```python
from build123d import *

# Parameters (mm, degrees)
PAD008_DEPTH = 2.8
FILLET001_R  = 0.4
POCKET_DEPTH = 2.801


with BuildPart() as part:
    # Sketch008 (on Face4 of ShapeBinder007) → Pad008 (new body)
    with BuildSketch(Plane(origin=(0, 20.1, 0), x_dir=(-1, 0, 0), z_dir=(0, 1, 0))):
        with BuildLine():
            Line((37.8, 63.2), (37.8, 60.4))
            Line((37.8, 60.4), (23.8, 60.4))
            ThreePointArc((23.8, 60.4), (23.4, 60), (23.8, 59.6))
            Line((23.8, 59.6), (37.8, 59.6))
            Line((37.8, 59.6), (37.8, -33.8))
            Line((37.8, -33.8), (23.8, -33.8))
            ThreePointArc((23.8, -33.8), (23.4, -34.2), (23.8, -34.6))
            Line((23.8, -34.6), (37.8, -34.6))
            Line((37.8, -34.6), (37.8, -37.4))
            Line((37.8, -37.4), (35.8, -38.15))
            Line((35.8, -38.15), (35.8, -37.4))
            Line((35.8, -37.4), (33, -37.4))
            Line((33, -39.4), (33, -37.4))
            Line((25.535898, -37.4), (33, -39.4))
            Line((-25.535898, -37.4), (25.535898, -37.4))
            Line((-33, -39.4), (-25.535898, -37.4))
            Line((-33, -37.4), (-33, -39.4))
            Line((-35.8, -37.4), (-33, -37.4))
            Line((-35.8, -38.15), (-35.8, -37.4))
            Line((-37.8, -37.4), (-35.8, -38.15))
            Line((-37.8, -37.4), (-37.8, -34.6))
            Line((-37.8, -34.6), (-23.8, -34.6))
            ThreePointArc((-23.8, -34.6), (-23.4, -34.2), (-23.8, -33.8))
            Line((-23.8, -33.8), (-37.8, -33.8))
            Line((-37.8, -33.8), (-37.8, 59.6))
            Line((-23.8, 59.6), (-37.8, 59.6))
            ThreePointArc((-23.8, 59.6), (-23.4, 60), (-23.8, 60.4))
            Line((-37.8, 60.4), (-23.8, 60.4))
            Line((-37.8, 60.4), (-37.8, 63.2))
            Line((-37.8, 63.2), (-35.8, 63.95))
            Line((-35.8, 63.95), (-35.8, 63.2))
            Line((-35.8, 63.2), (-33, 63.2))
            Line((-33, 65.2), (-33, 63.2))
            Line((-25.535898, 63.2), (-33, 65.2))
            Line((25.535898, 63.2), (-25.535898, 63.2))
            Line((33, 65.2), (25.535898, 63.2))
            Line((33, 63.2), (33, 65.2))
            Line((35.8, 63.2), (33, 63.2))
            Line((35.8, 63.95), (35.8, 63.2))
            Line((37.8, 63.2), (35.8, 63.95))
        make_face()
    extrude(amount=-PAD008_DEPTH)

    # Fillet001
    fillet001_edges = [part.edges().sort_by_distance(p)[0] for p in [
        (-33, 18.7, 65.2),
        (-37.8, 18.7, 63.2),
        (-37.8, 18.7, 60.4),
        (-37.8, 18.7, 59.6),
        (-37.8, 18.7, -33.8),
        (-37.8, 18.7, -34.6),
        (-37.8, 18.7, -37.4),
        (-33, 18.7, -39.4),
        (33, 18.7, 65.2),
        (37.8, 18.7, 63.2),
        (37.8, 18.7, 60.4),
        (37.8, 18.7, 59.6),
        (37.8, 18.7, -33.8),
        (37.8, 18.7, -34.6),
        (37.8, 18.7, -37.4),
        (33, 18.7, -39.4),
    ]]
    fillet(fillet001_edges, radius=FILLET001_R)

    # Sketch029 (on Face2 of Fillet001) → Pocket (cut, through all)
    with BuildSketch(Plane(origin=(0, 20.1, 0), x_dir=(-1, 0, 0), z_dir=(0, 1, 0))):
        with BuildLine():
            Line((-11.39, -34.8), (11.39, -34.8))
            ThreePointArc((11.39, -34.8), (13.043156, -34.001173), (13.444572, -32.209549))
            ThreePointArc((13.444577, -19.790431), (12.728234, -25.99999), (13.444572, -32.209549))
            ThreePointArc((13.444577, -19.790431), (13.04315, -17.998819), (11.39, -17.2))
            Line((11.39, -17.2), (-11.39, -17.2))
            ThreePointArc((-11.39, -17.2), (-13.04315, -17.998819), (-13.444577, -19.790431))
            ThreePointArc((-13.444577, -32.209569), (-12.728234, -26), (-13.444577, -19.790431))
            ThreePointArc((-13.444577, -32.209569), (-13.04315, -34.001181), (-11.39, -34.8))
        make_face()
        with BuildLine():
            ThreePointArc((-15.62035, -17.781737), (-16.614302, -17.232088), (-17.156126, -18.230327))
            ThreePointArc((-17.156126, -33.769673), (-16.013455, -26), (-17.156126, -18.230327))
            ThreePointArc((-17.156126, -33.769673), (-16.614302, -34.767912), (-15.62035, -34.218263))
            ThreePointArc((-15.62035, -34.218263), (-14.477584, -26), (-15.62035, -17.781737))
        make_face()
        with BuildLine():
            ThreePointArc((17.156126, -18.230327), (16.614302, -17.232088), (15.62035, -17.781737))
            ThreePointArc((15.62035, -17.781737), (14.477584, -26), (15.62035, -34.218263))
            ThreePointArc((15.62035, -34.218263), (16.614302, -34.767912), (17.156126, -33.769673))
            ThreePointArc((17.156126, -18.230327), (16.013455, -26), (17.156126, -33.769673))
        make_face()
    extrude(amount=-POCKET_DEPTH, mode=Mode.SUBTRACT)


solid = part.part
```
Can you work these out from the model? Positions are in its coordinate system, mm. A direction names the side the tool comes from. Coordinates: 2 decimals unless noted, no trailing zeros. Order: outer loops, then holes, each group sorted by start corner. A loop starts at its lowest first (then second) coordinate and runs counter-clockwise, first axis right, second up.
1. I'm going to push flat-ended pins straight in: pin 1 (0.8 mm diameter, centred on x = -34, y = 19, fed in from +Z); pin 2 (0.8 mm diameter, centred on x = 32, y = 18, fed in from -Z); pin 3 (1.6 mm diameter, centred on y = 18.5, z = -38, fed in from -X). Where does each tip first touch, or does it pass through?
2. If we section it at A-A (x = 9): Please give me the cut outline in (y, z), then the cut area to 3 significant figures.
3. If we section it at D-D (x = 19): Please give me the cut outline in (y, z).
4. If we section it at B-B (x = 27): Please give me the cut outline in (y, z).
5. Thinking about a two-plate mould opening in X: for faces 5 (the face through (-37.8, 19, -36)), 6 (the face through (-31, 19, 60.4)), 7 (the face through (-28.97, 18.72, -38.32)), 8 (the face through (0, 19, -37.4)), which applies, +X half, -X half, draft (parallel to the pull), parting line (faces both ways), or undercut?
6. I need wall thicknesses on line 1 (Z direction, x = -34, y = 18.25); line 2 (X direction, y = 17.95, z = -25); line 3 (Z direction, x = 3.5, y = 19.15). Which ranges of each line are inside material? Lowest first, please.
7. If we section it at C-C (y = 17.85): Give the number of separate pieces and of enclosed holes in the cut face, then the cut area to 3 significant figures.
8. For faces 1 (the face through (-34, 19, -37.4)), 2 (the face through (34, 19, 63.2)), 3 (the face through (-14.478, 18.72, -25.883)), 4 (the face through (-31, 19, -33.8)), which set-ups out of +Z, -Z, +X, -X, +Y, -Y let a thin tool reach every point of the face, with its end or its side?
Entries:
1. pin 1: stops at z = 63.2
1. pin 2: stops at z = -39.24
1. pin 3: stops at x = -37.79
2. outline: (17.3, -37.4) - (20.1, -37.4) - (20.1, -34.8) - (17.3, -34.8) - close; (17.3, -17.2) - (20.1, -17.2) - (20.1, 63.2) - (17.3, 63.2) - close
2. area: 232 mm2
3. outline: (17.3, -37.4) - (20.1, -37.4) - (20.1, 63.2) - (17.3, 63.2) - close
4. outline: (17.3, -37.79) - (20.1, -37.79) - (20.1, -34.6) - (17.3, -34.6) - close; (17.3, -33.8) - (20.1, -33.8) - (20.1, 59.6) - (17.3, 59.6) - close; (17.3, 60.4) - (20.1, 60.4) - (20.1, 63.59) - (17.3, 63.59) - close
5. face 5: -X half
5. face 6: draft
5. face 7: undercut
5. face 8: undercut
6. line 1: z = -37.4 to -34.6, -33.8 to 59.6, 60.4 to 63.2
6. line 2: x = -37.8 to -16.03, -14.49 to -12.75, 12.75 to 14.49, 16.03 to 37.8
6. line 3: z = -37.4 to -34.8, -17.2 to 63.2
7. separate pieces: 1
7. enclosed holes: 3
7. area: 7,080 mm2
8. face 1: -Z, +Y, -Y
8. face 2: +Z, +Y, -Y
8. face 3: +Y, -Y
8. face 4: -X, +Y, -Y
